The model under review builds one solid part; all positions refer to its coordinate system, in mm. Face numbers are marked on the shaded views. Coordinates: 2 decimals unless noted, no trailing zeros. Loops run counter-clockwise (first coordinate to the right, second up) from the corner with the lowest first, then second, coordinate; pieces in that order, holes last. Notation, with made-up numbers: (20.25, -12.75) - (77.25, -12.75) arc R30 ccw to (77.25, 18.25) - close; hole circle Ø4 at (3.5, 37). An arc over 180 degrees is marked (long way). Use a Markdown table: item, result. Add a question column.
1) Add section C-C, the plane z = 5.5. Give the boundary of the cut face in (x, y), and give its area (3 significant figures).
2) Add section D-D, the plane y = 6. Give the number of separate pieces and of enclosed holes in the cut face, and give its area (3 significant figures).
3) Clearance check with flat-ended pins moving along their axes: pin 1 (0.6 mm diameter, centred on x = 16, z = 1, fed in from +Y); pin 2 (1 mm diameter, centred on x = -16, z = 1, fed in from +Y); pin 3 (0.6 mm diameter, centred on y = 17.5, z = 1, fed in from -X). State where each tip first meets the part, or that it passes through.
4) The part is to be moulded in two halves that separate along X. For the marked faces 1 and 2, say which applies: pulls with the +X half, pulls with the -X half, needs draft (parallel to the pull), parting line crosses it, or undercut.
5) Add section A-A, the plane y = 0. Give the boundary of the cut face in (x, z).
```python
from build123d import *

# Parameters (mm, degrees)
SKETCH_2_R      = 22
SKETCH_2_R_2    = 11
EXTRUDE_1_DEPTH = 2


with BuildPart() as part:
    # Эскиз2 → Бобышка-Вытянуть1 (new body)
    with BuildSketch(Plane.XY):
        Circle(SKETCH_2_R)
        with BuildLine():
            Line((12.961481397, -1), (19.974984355, -1))
            ThreePointArc((19.974984355, -1), (14.142135624, -14.142135624), (1, -19.974984355))
            Line((1, -19.974984355), (1, -12.961481397))
            ThreePointArc((1, -12.961481397), (9.192388155, -9.192388155), (12.961481397, -1))
        make_face(mode=Mode.SUBTRACT)
        with BuildLine():
            Line((19.974984355, 1), (12.961481397, 1))
            ThreePointArc((12.961481397, 1), (9.192388155, 9.192388155), (1, 12.961481397))
            Line((1, 12.961481397), (1, 19.974984355))
            ThreePointArc((1, 19.974984355), (14.142135624, 14.142135624), (19.974984355, 1))
        make_face(mode=Mode.SUBTRACT)
        with BuildLine():
            Line((-1, 19.974984355), (-1, 12.961481397))
            ThreePointArc((-1, 12.961481397), (-9.192388155, 9.192388155), (-12.961481397, 1))
            Line((-12.961481397, 1), (-19.974984355, 1))
            ThreePointArc((-19.974984355, 1), (-14.142135624, 14.142135624), (-1, 19.974984355))
        make_face(mode=Mode.SUBTRACT)
        with BuildLine():
            Line((-19.974984355, -1), (-12.961481397, -1))
            ThreePointArc((-12.961481397, -1), (-9.192388155, -9.192388155), (-1, -12.961481397))
            Line((-1, -12.961481397), (-1, -19.974984355))
            ThreePointArc((-1, -19.974984355), (-14.142135624, -14.142135624), (-19.974984355, -1))
        make_face(mode=Mode.SUBTRACT)
        Circle(SKETCH_2_R_2, mode=Mode.SUBTRACT)
    extrude(amount=EXTRUDE_1_DEPTH)

    # Эскиз4 → Повернуть1 (revolve)
    with BuildSketch(Plane(origin=(0, 0, 0), x_dir=(1, 0, 0), z_dir=(0, 1, 0)), mode=Mode.PRIVATE) as revolve_1_sk:
        Polygon((11, -2), (8, -8), (9, -8), (12.961481397, -2), align=None)
        Polygon((14, -8), (19.974984355, -2), (22, -2), (15, -8), align=None)
    revolve(revolve_1_sk.sketch.rotate(Axis((0, 0, -0.4), (0, 0, 1)), 180), axis=Axis((0, 0, -0.4), (0, 0, 1)))


solid = part.part
```
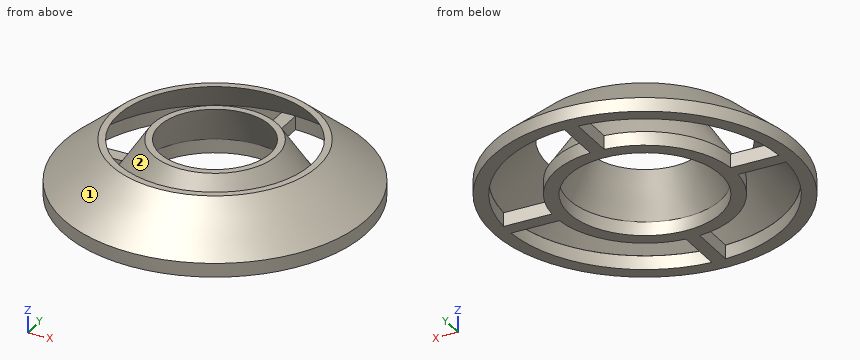
From the geometry:
| question | item | result |
|---|---|---|
| 1 | outline | circle Ø35.83 at (0, 0); circle Ø21.3 at (0, 0); hole circle Ø32.98 at (0, 0); hole circle Ø18.5 at (0, 0) |
| 1 | area | 242 mm^2 |
| 2 | separate pieces | 4 |
| 2 | enclosed holes | 0 |
| 2 | area | 58.9 mm^2 |
| 3 | pin 1 | stops at y = 15.41 |
| 3 | pin 2 | stops at y = 15.61 |
| 3 | pin 3 | stops at x = -13.72 |
| 4 | face 1 | parting line crosses it |
| 4 | face 2 | undercut |
| 5 | outline | (-22, 0) - (-11, 0) - (-11, 2) - (-8, 8) - (-9, 8) - (-12.96, 2) - (-19.97, 2) - (-14, 8) - (-15, 8) - (-22, 2) - close; (8, 8) - (11, 2) - (11, 0) - (22, 0) - (22, 2) - (15, 8) - (14, 8) - (19.97, 2) - (12.96, 2) - (9, 8) - close |
